Part model, mm, in its own coordinate system. A direction names the side the tool comes from. Round coordinates to 2 decimals unless told otherwise and drop trailing zeros. Order: outer loops, then holes, each group sorted by start corner. A loop starts at its lowest first (then second) coordinate and runs counter-clockwise, first axis right, second up. Notation, with made-up numbers: M 54.5,-31 L 100.5,-31 A8 cw 100.5,-19 Z; hole C -34.5,30.5 d5. An arc over 180 degrees is marked long. Write each question's results on one line, items separated by ' | '. Start each with the question number.
1. Which spindle directions (+Z, -Z, +X, -X, +Y, -Y) get a long thin tool onto all of the face, cutting with end or side? Do faces 1 (the face through (0, 59, 2)), 2 (the face through (62, 61, 3.5)), 3 (the face through (7, 61, 3.5)). Say none if no direction does.
2. Band-saw the part on D-D, the plane z = 8.5. List the corners of the cut face in (x, y), then the cut area to 3 significant figures.
3. Band-saw the part on B-B, the plane x = 7.5. List the corners of the cut face in (y, z).
4. Drop flat-ended pins along their axis: pin 1 Ø5 at (y, z) = (26, 4.5) entering from +X; pin 2 Ø2 at (y, z) = (75, 8.5) entering from -X; pin 3 Ø1 at (x, y) = (52.5, 90) entering from +Z; pin 4 Ø16.5 at (x, y) = (7, 77) entering from +Z. Give the stop position or say it passes through.
5. Probe L1, parallel to Z at x = 60.5, y = 95.5; L2, parallel to X at y = 10.5, z = 6.75; L3, parallel to Z at x = 52, y = 104.5. List the from-to ranges inside material, lowest first. Write a range as [from, to].
```python
from build123d import *

# Parameters (mm, degrees)
SKETCH_1_W      = 70
SKETCH_1_H      = 120
EXTRUDE_1_DEPTH = 3.5
SKETCH_2_W      = 20.2
SKETCH_2_H      = 120
EXTRUDE_2_DEPTH = 10
FILLET_1_R      = 10
FILLET_2_R      = 20


with BuildPart() as part:
    # ｽｹｯﾁ1 → ﾎﾞｽ - 押し出し1 (new body)
    with BuildSketch(Plane.XY):
        with Locations((35, 60)):
            Rectangle(SKETCH_1_W, SKETCH_1_H)
    extrude(amount=EXTRUDE_1_DEPTH)

    # ｽｹｯﾁ2 → ﾎﾞｽ - 押し出し2 (add)
    with BuildSketch(Plane.XY.offset(3.5)):
        with Locations((35, 60)):
            Rectangle(SKETCH_2_W, SKETCH_2_H)
    extrude(amount=EXTRUDE_2_DEPTH)

    # ﾌｨﾚｯﾄ1
    fillet_1_edges = [part.edges().sort_by_distance(p)[0] for p in [
        (24.9, 60, 3.5),
        (45.1, 60, 3.5),
    ]]
    fillet(fillet_1_edges, radius=FILLET_1_R - 0.0001)  # a hair under: the kernel refuses the full size

    # ﾌｨﾚｯﾄ2
    fillet_2_edges = [part.edges().sort_by_distance(p)[0] for p in [
        (70, 120, 1.75),
        (70, 0, 1.75),
        (0, 0, 1.75),
        (0, 120, 1.75),
    ]]
    fillet(fillet_2_edges, radius=FILLET_2_R)


solid = part.part
```
Solution:
1) face 1: +Z, -Z, -X, +Y, -Y | face 2: +Z, +X, +Y, -Y | face 3: +Z, -X, +Y, -Y
2) outline: M 23.56,0 L 46.44,0 L 46.44,120 L 23.56,120 Z | area: 2,750 mm^2
3) outline: M 4.39,0 L 115.61,0 L 115.61,3.5 L 4.39,3.5 Z
4) pin 1: x = 70 | pin 2: x = 22.9 | pin 3: z = 3.99 | pin 4: z = 3.51
5) L1: [0, 3.5] | L2: [22.28, 47.72] | L3: [0, 3.99]
